from build123d import *

# Parameters (mm, degrees)
FILLET1_SIZE   = 4.9
FILLET1_SIZE_2 = 1.5


with BuildPart() as part:
    # Sketch1 → Revolve1 (revolve)
    with BuildSketch(Plane(origin=(0, 0, 0), x_dir=(0, 0, -1), z_dir=(1, 0, 0)), mode=Mode.PRIVATE) as revolve1_sk:
        Polygon((3, -1), (0, -1), (0, -27), (2.4, -27), (2.4, -34), (3, -34), align=None)
        Polygon((5, 1), (0, 1), (0, -1), (3, -1), (5, -1), align=None)
    revolve(revolve1_sk.sketch.rotate(Axis((0, 1, 0), (0, -1, 0)), 180), axis=Axis((0, 1, 0), (0, -1, 0)))

    # Fillet1
    # an asymmetric fillet: 4.9, 1.5 mm, written as the material it takes off along each edge
    with BuildSketch(Plane(origin=(0, 1, 0), x_dir=(0, 0, 1), z_dir=(1, 0, 0))) as fillet1_piece_1:
        with BuildLine():
            Bezier((5 - FILLET1_SIZE, 0), (5, 0), (5, FILLET1_SIZE_2), weights=[1, 0.707106781, 1])
            Line((5, FILLET1_SIZE_2), (5, 0))
            Line((5, 0), (5 - FILLET1_SIZE, 0))
        make_face()
    revolve(axis=Axis((0, 1, 0), (0, -1, 0)), mode=Mode.SUBTRACT)


solid = part.part
Design review of the part built by this model. Coordinates are the model's own, in mm. Give positions to 0.01 mm unless a question says otherwise; leave off trailing zeros. Loops run counter-clockwise (first coordinate to the right, second up) from the corner with the lowest first, then second, coordinate; pieces in that order, holes last. Notation, with made-up numbers: (51.5, 46.25) - (107.5, 46.25) arc R17 cw to (107.5, 58.25) - close; hole circle Ø10 at (-9.75, 41). An arc over 180 degrees is marked (long way). Use CSV: the item, a comma, the result in double quotes. Start each with the question number.
1. Draft analysis for pull direction Z (two halves, no side actions). For faces 1 (the cylindrical face through (-0.22, -0.746, -4.995)), 2 (the flat face through (0, -27, 0)), 3 (the flat face through (3.3, -1, 0.1)), state which applies: released by +Z, released by -Z, zero draft, split by the parting line, or undercut.
2. Add section A-A (y = -5). State the section outline as (x, z) points, plus the area to 3 significant figures.
3. Wall thickness on L1, parallel to X at y = -30, z = 0; L2, parallel to Y at x = -0.25, z = 0; L3, parallel to X at y = -18, z = 0: over which ranges is each line inside the solid? List them lowest first.
4. Insertion check: P1, Ø1.5, axis at y = -17, z = 4, coming from the +X side; P2, Ø6, axis at y = -12.5, z = 2.5, coming from the -X side; P3, Ø3, axis at x = 0.5, z = 0, coming from the -Y side; P4, Ø3, axis at x = -2, y = -17.5, coming from the +Z side. Each pin has a flat end and moves straight along its axis. Give the tip position at first contact, or say it passes through.
Results found:
1,face 1,"split by the parting line"
1,face 2,"undercut"
1,face 3,"zero draft"
2,outline,"circle Ø6 at (0, 0)"
2,area,"28.3 mm²"
3,L1,"x = -3 to -2.4, 2.4 to 3"
3,L2,"y = -27 to 1"
3,L3,"x = -3 to 3"
4,P1,"passes through"
4,P2,"stops at x = -3"
4,P3,"stops at y = -27"
4,P4,"stops at z = 2.96"
